from build123d import *

# Parameters (mm, degrees)
SKETCH1_R           = 3.175
BOSS_EXTRUDE1_DEPTH = 11.43
SKETCH2_W           = 161.464261653
SKETCH2_H           = 32
BOSS_EXTRUDE2_DEPTH = 12.7
SKETCH5_R           = 3.175
BOSS_EXTRUDE3_DEPTH = 11.43
SKETCH6_W           = 77
SKETCH6_H           = 11.5
CUT_EXTRUDE1_DEPTH  = 7.5
BOSS_EXTRUDE4_DEPTH = 19.05
CUT_EXTRUDE3_DEPTH  = 30.48
BOSS_EXTRUDE5_DEPTH = 25.4
SKETCH7_W           = 12
SKETCH7_H           = 11.5
CUT_EXTRUDE4_DEPTH  = 50.8
SKETCH7_5_W         = 12
SKETCH7_5_H         = 11.5
CUT_EXTRUDE5_DEPTH  = 50.8
SKETCH16_W          = 12.7
SKETCH16_H          = 32
CUT_EXTRUDE6_DEPTH  = 8.89
SKETCH17_R          = 1
CUT_EXTRUDE7_DEPTH  = 4.299778595
SKETCH18_W          = 12.7
SKETCH18_H          = 32
CUT_EXTRUDE8_DEPTH  = 19.05
CUT_EXTRUDE9_DEPTH  = 3.81


with BuildPart() as part:
    # Sketch1 → Boss-Extrude1 (new body)
    with BuildSketch(Plane.XY):
        with BuildLine():
            Line((-47.217391304, 7.923913043), (130.582608696, 7.923913043))
            ThreePointArc((130.582608696, 7.923913043), (146.582608696, -8.076086957), (130.582608696, -24.076086957))
            Line((130.582608696, -24.076086957), (-47.217391304, -24.076086957))
            ThreePointArc((-47.217391304, -24.076086957), (-63.217391304, -8.076086957), (-47.217391304, 7.923913043))
        make_face()
        with Locations((-47.217391304, -8.076086957)):
            Circle(SKETCH1_R, mode=Mode.SUBTRACT)
        with Locations((130.582608696, -8.076086957)):
            Circle(SKETCH1_R, mode=Mode.SUBTRACT)
    extrude(amount=BOSS_EXTRUDE1_DEPTH)

    # Sketch2 → Boss-Extrude2 (add)
    with BuildSketch(Plane.XY.offset(11.43)):
        with Locations((41.59547787, -8.076086957)):
            Rectangle(SKETCH2_W, SKETCH2_H)
    extrude(amount=BOSS_EXTRUDE2_DEPTH)

    # Sketch5 → Boss-Extrude3 (add)
    with BuildSketch(Plane.XY.offset(24.13)):
        with BuildLine():
            Line((-47.217391304, 7.923913043), (130.582608696, 7.923913043))
            ThreePointArc((130.582608696, 7.923913043), (146.582608696, -8.076086957), (130.582608696, -24.076086957))
            Line((130.582608696, -24.076086957), (-47.217391304, -24.076086957))
            ThreePointArc((-47.217391304, -24.076086957), (-63.217391304, -8.076086957), (-47.217391304, 7.923913043))
        make_face()
        with Locations((-47.217391304, -8.076086957)):
            Circle(SKETCH5_R, mode=Mode.SUBTRACT)
        with Locations((130.582608696, -8.076086957)):
            Circle(SKETCH5_R, mode=Mode.SUBTRACT)
    extrude(amount=BOSS_EXTRUDE3_DEPTH)

    # Sketch6 → Cut-Extrude1 (cut)
    with BuildSketch(Plane(origin=(0, 7.923913043, 0), x_dir=(1, 0, 0), z_dir=(0, 1, 0))):
        with Locations((41.682608696, -17.78)):
            Rectangle(SKETCH6_W, SKETCH6_H)
    extrude(amount=-CUT_EXTRUDE1_DEPTH, mode=Mode.SUBTRACT)

    # Sketch10 → Boss-Extrude4 (add)
    with BuildSketch(Plane.XY.offset(35.56)):
        with BuildLine():
            Line((-34.517391304, -20.776086957), (-57.377391304, -20.776086957))
            ThreePointArc((-57.377391304, -20.776086957), (-59.173442529, -20.032138181), (-59.917391304, -18.236086957))
            Line((-59.917391304, -18.236086957), (-59.917391304, 2.083913043))
            ThreePointArc((-59.917391304, 2.083913043), (-59.173442529, 3.879964268), (-57.377391304, 4.623913043))
            Line((-57.377391304, 4.623913043), (-34.517391304, 4.623913043))
            Line((-34.517391304, 4.623913043), (-21.817391304, 4.623913043))
            Line((-21.817391304, 4.623913043), (-21.817391304, -20.776086957))
            Line((-21.817391304, -20.776086957), (-34.517391304, -20.776086957))
        make_face()
    extrude(amount=BOSS_EXTRUDE4_DEPTH)

    # Sketch14 → Cut-Extrude3 (cut)
    with BuildSketch(Plane(origin=(0, 4.623913043, 0), x_dir=(1, 0, 0), z_dir=(0, 1, 0))):
        with BuildLine():
            Line((-59.917391304, -35.56), (-29.183391304, -35.56))
            ThreePointArc((-29.183391304, -35.56), (-29.434604535, -44.304535578), (-35.79555952, -50.310221405))
            Line((-35.79555952, -50.310221405), (-59.917391304, -50.310221405))
            Line((-59.917391304, -50.310221405), (-59.917391304, -35.56))
        make_face()
    extrude(amount=-CUT_EXTRUDE3_DEPTH, mode=Mode.SUBTRACT)

    # Sketch15 → Boss-Extrude5 (add)
    with BuildSketch(Plane.XZ.offset(20.776086957)):
        Polygon((-21.817391304, 35.56), (5.46367495, 35.56), (-21.817391304, 54.61), align=None)
    extrude(amount=-BOSS_EXTRUDE5_DEPTH)

    # Sketch7 → Cut-Extrude4 (cut)
    with BuildSketch(Plane(origin=(0, 0.423913043, 0), x_dir=(1, 0, 0), z_dir=(0, 1, 0))):
        with Locations((74.182608696, -17.78)):
            Rectangle(SKETCH7_W, SKETCH7_H)
    extrude(amount=-CUT_EXTRUDE4_DEPTH, mode=Mode.SUBTRACT)

    # Sketch7<5> → Cut-Extrude5 (cut)
    with BuildSketch(Plane(origin=(0, 0.423913043, 0), x_dir=(1, 0, 0), z_dir=(0, 1, 0))):
        with Locations((9.182608696, -17.78)):
            Rectangle(SKETCH7_5_W, SKETCH7_5_H)
    extrude(amount=-CUT_EXTRUDE5_DEPTH, mode=Mode.SUBTRACT)

    # Sketch16 → Cut-Extrude6 (cut)
    with BuildSketch(Plane.ZY.offset(39.136652957)):
        with Locations((17.78, -8.076086957)):
            Rectangle(SKETCH16_W, SKETCH16_H)
    extrude(amount=-CUT_EXTRUDE6_DEPTH, mode=Mode.SUBTRACT)

    # Sketch17 → Cut-Extrude7 (cut)
    with BuildSketch(Plane(origin=(0, 0, 50.310221405), x_dir=(-1, 0, 0), z_dir=(0, 0, -1))):
        with Locations((38.327391304, 0.813913043)):
            Circle(SKETCH17_R)
        with Locations((56.107391304, 0.813913043)):
            Circle(SKETCH17_R)
        with Locations((56.107391304, -16.966086957)):
            Circle(SKETCH17_R)
        with Locations((38.327391304, -16.966086957)):
            Circle(SKETCH17_R)
    extrude(amount=-CUT_EXTRUDE7_DEPTH, mode=Mode.SUBTRACT)

    # Sketch18 → Cut-Extrude8 (cut)
    with BuildSketch(Plane(origin=(122.327608696, 0, 0), x_dir=(0, 0, -1), z_dir=(1, 0, 0))):
        with Locations((-17.78, -8.076086957)):
            Rectangle(SKETCH18_W, SKETCH18_H)
    extrude(amount=-CUT_EXTRUDE8_DEPTH, mode=Mode.SUBTRACT)

    # Sketch19 → Cut-Extrude9 (cut)
    with BuildSketch(Plane(origin=(0, 0, 0), x_dir=(-1, 0, 0), z_dir=(0, 0, -1))):
        Polygon((-130.582608696, -1.47697338), (-136.297608696, -4.776530168), (-136.297608696, -11.375643745), (-130.582608696, -14.675200533), (-124.867608696, -11.375643745), (-124.867608696, -4.776530168), align=None)
    extrude(amount=-CUT_EXTRUDE9_DEPTH, mode=Mode.SUBTRACT)


solid = part.part
The listing builds one solid part. Answer for the finished solid, in the listing's coordinates (mm). A direction names the side the tool comes from. Give positions to 0.01 mm unless a question says otherwise; leave off trailing zeros. Order: outer loops, then holes, each group sorted by start corner. A loop starts at its lowest first (then second) coordinate and runs counter-clockwise, first axis right, second up. Notation, with made-up numbers: (24.25, 81.25) -> (65.25, 81.25) arc R23 cw to (65.25, 110.25) -> close; hole circle Ø3 at (18.5, -26.75). An arc over 180 degrees is marked (long way). Put each result on its own line as item: value.
Item 1: A cutting plane is placed at D-D on z = 30.5. Give the vertices of the cut face in (x, y) (3 decimals), plus the area to 3 significant figures.
Established:
outline: (-47.217, -24.076) -> (130.583, -24.076) arc R16 ccw to (130.583, 7.924) -> (-47.217, 7.924) arc R16 ccw to start; hole circle Ø6.35 at (-47.217, -8.076); hole circle Ø6.35 at (130.583, -8.076)
area: 6,430 mm^2
Item 2: Given P1, Ø1.1, axis at y = -7, z = 1, coming from the +X side; P2, Ø4, axis at y = -10, z = 19.5, coming from the -X side; P3, Ø6, axis at x = 111, y = -16, coming from the +Z side; P4, Ø4, axis at x = 130.58, y = -8.08, coming from the +Z side, each flat-ended and moving along its own axis, determine where each tip first touches the part or whether it passes through.
Established:
P1: stops at x = 146.57
P2: stops at x = -30.25
P3: stops at z = 35.56
P4: passes through
Item 3: For faces 5 (the face through (3.183, -8, 18)), 6 (the face through (-63.214, -8.428, 29.765)), 7 (the face through (41, 3, 12.03)), 8 (the face through (-43, -8, 11.43)), determine the directions among +Z, -Z, +X, -X, +Y, -Y from which every point of the face is accessible in a straight line to the end or side of a thin tool.
Established:
face 5: +Y, -Y
face 6: -Z, -X
face 7: +Y
face 8: -X, +Y, -Y
Item 4: Straight lines are drawn through the part: line 1 (X direction, y = -23, z = 17); line 2 (Z direction, x = -32, y = -23); line 3 (Z direction, x = 65, y = -1). For each, find the intervals that lie inside material, in ascending order.
Established:
line 1: x = -30.25 to 3.18, 15.18 to 68.18, 80.18 to 103.28
line 2: z = 0 to 11.43, 24.13 to 35.56
line 3: z = 0 to 35.56
Item 5: For a pull along Z with two mould halves and no side action, classify faces 1 (the face through (132, -5, 3.81)), 2 (the face through (-29.384, -7.898, 44.19)), 3 (the face through (-30.247, -8, 18)), 4 (the face through (146.58, -7.72, 5.63)) as released by +Z, released by -Z, zero draft, split by the parting line, or undercut.
Established:
face 1: released by -Z
face 2: undercut
face 3: undercut
face 4: zero draft
Item 6: A cutting plane is placed at C-C on x = 8.5. Give the vertices of the cut face in (y, z), plus the area to 3 significant figures.
Established:
outline: (-24.08, 0) -> (7.92, 0) -> (7.92, 12.03) -> (-24.08, 12.03) -> close; (-24.08, 23.53) -> (7.92, 23.53) -> (7.92, 35.56) -> (-24.08, 35.56) -> close
area: 770 mm^2
Item 7: A cutting plane is placed at A-A on z = 19. Give the vertices of the cut face in (x, y).
Established:
outline: (-30.25, -24.08) -> (3.18, -24.08) -> (3.18, 7.92) -> (-30.25, 7.92) -> close; (15.18, -24.08) -> (68.18, -24.08) -> (68.18, 0.42) -> (15.18, 0.42) -> close; (80.18, -24.08) -> (103.28, -24.08) -> (103.28, 7.92) -> (80.18, 7.92) -> close
Item 8: A cutting plane is placed at B-B on x = 106. Give the vertices of the cut face in (y, z), plus the area to 3 significant figures.
Established:
outline: (-24.08, 0) -> (7.92, 0) -> (7.92, 11.43) -> (-24.08, 11.43) -> close; (-24.08, 24.13) -> (7.92, 24.13) -> (7.92, 35.56) -> (-24.08, 35.56) -> close
area: 732 mm^2
